Answer from the drawing. Dimensions are ordinates in mm from the lowest x, y and z of the part. A direction names the side the tool comes from. Coordinates: 2 decimals unless noted, no trailing zeros. Write each loop counter-clockwise with the first axis right and the second up, starting at its lowest first coordinate (ties: lowest second). Pieces come first, ordered by that corner, then holes.
(1) Given pin 1 (20 mm diameter, centred on y = 75, z = 85, fed in from +X); pin 2 (2 mm diameter, centred on x = 34.5, z = 83, fed in from +Y); pin 3 (10 mm diameter, centred on y = 75, z = 50, fed in from -X), each flat-ended and moving along its own axis, determine where each tip first touches the part or whether it passes through.
(2) Which of the six approach directions +Z, -Z, +X, -X, +Y, -Y give full straight-line access (tool end or side, diameter ignored) to the marked faces 4 and 5?
(3) Section D-D on x = 21 is taken. Write down the section's boundary in (y, z), then the cut area to 3 significant figures.
(4) The mould has two halves that part along X. Classify the marked faces 1, 2 and 3: +X half, -X half, draft (parallel to the pull), parting line (faces both ways), or undercut.
(5) Find the intervals of material crossed by probe 1 along Y at (x, z) = (6, 85); probe 2 along X at (y, z) = (7.5, 50); probe 3 along Y at (x, z) = (68, 78.5), in increasing order.
(6) Section B-B on y = 7.5 is taken. Write down the section's boundary in (x, z), then the cut area to 3 significant figures.
(7) Section A-A on z = 50 is taken. Write down the section's boundary in (x, y), then the cut area to 4 significant figures.
(8) Section C-C on z = 85 is taken. Write down the section's boundary in (x, y).
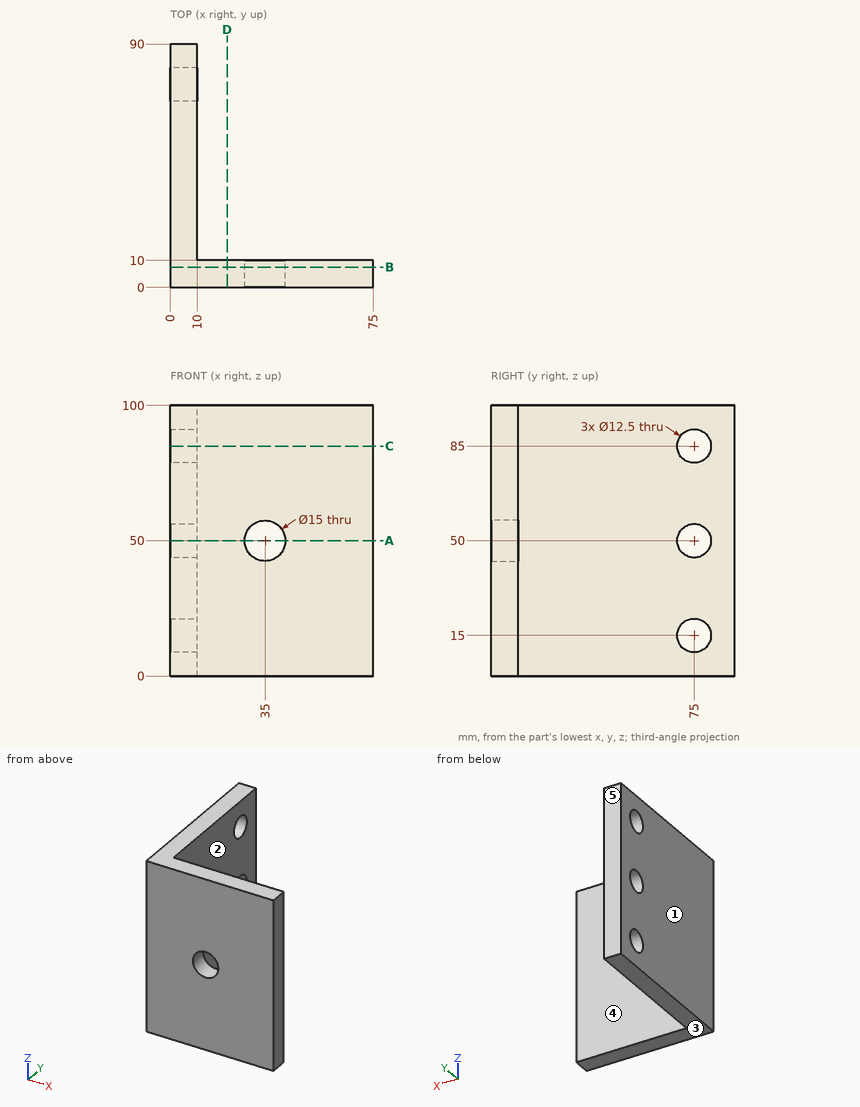
Response:
1. pin 1: stops at x = 10
1. pin 2: stops at y = 10
1. pin 3: passes through
2. face 4: +Z, -Z, +X, +Y
2. face 5: +Z, -Z, +X, -X, +Y
3. outline: (0, 0) - (10, 0) - (10, 100) - (0, 100) - close
3. area: 1,000 mm2
4. face 1: -X half
4. face 2: +X half
4. face 3: draft
5. probe 1: y = 0 to 68.75, 81.25 to 90
5. probe 2: x = 0 to 27.5, 42.5 to 75
5. probe 3: y = 0 to 10
6. outline: (0, 0) - (75, 0) - (75, 100) - (0, 100) - close; hole circle Ø15 at (35, 50)
6. area: 7,320 mm2
7. outline: (0, 0) - (27.5, 0) - (27.5, 10) - (10, 10) - (10, 68.75) - (0, 68.75) - close; (0, 81.25) - (10, 81.25) - (10, 90) - (0, 90) - close; (42.5, 0) - (75, 0) - (75, 10) - (42.5, 10) - close
7. area: 1,275 mm2
8. outline: (0, 0) - (75, 0) - (75, 10) - (10, 10) - (10, 68.75) - (0, 68.75) - close; (0, 81.25) - (10, 81.25) - (10, 90) - (0, 90) - close
